The listing builds one solid part. Answer for the finished solid, in the listing's coordinates (mm). Face numbers are marked on the shaded views. Round coordinates to 2 decimals unless told otherwise and drop trailing zeros. Order: outer loops, then holes, each group sorted by start corner. A loop starts at its lowest first (then second) coordinate and runs counter-clockwise, first axis right, second up. Notation, with made-up numbers: (22, -5.5) - (51, -5.5) arc R18 ccw to (51, 21.5) - close; hole circle Ø7 at (51, -30.75). An arc over 180 degrees is marked (long way). One line per item, written item: value. Start each with the question number.
1. Section A-A, the plane z = 0 is taken. Give the vertices of the cut face in (x, y), then the cut area to 3 significant figures.
2. Straight lines are drawn through the part: line 1 (X direction, y = 0.2, z = 0.25); line 2 (Z direction, x = 10, y = 1.25); line 3 (X direction, y = 1.8, z = 10). For each, find the intervals that lie inside material, in ascending order.
3. Section C-C, the plane z = -10 is taken. Give the vertices of the cut face in (x, y), then the cut area to 3 significant figures.
4. Section B-B, the plane x = 10 is taken. Give the vertices of the cut face in (y, z), then the cut area to 3 significant figures.
5. Section D-D, the plane y = 0.5 is taken. Give the vertices of the cut face in (x, z).
6. Flat-ended cylindrical pins translate along their axes: P1, Ø1.3, axis at x = 10, z = 0, coming from the -Y side; P2, Ø0.6, axis at y = 1, z = 8.5, coming from the -X side. Find the tip coordinate at first contact, or state that the pin passes through.
7. For a pull along Z with two mould halves and no side action, classify the marked faces 1, 2, 3 and 4 as released by +Z, released by -Z, zero draft, split by the parting line, or undercut.
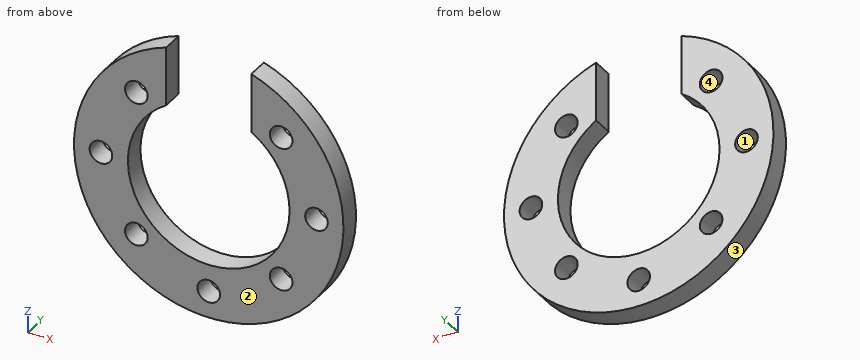
from build123d import *

# Parameters (mm, degrees)
SKETCH1_R           = 12.5
SKETCH1_R_2         = 7.5
BOSS_EXTRUDE1_DEPTH = 2
SKETCH2_R           = 1.05
CUT_EXTRUDE1_DEPTH  = 5
CIRPATTERN1_COUNT   = 3
CIRPATTERN1_ANGLE   = 180
SKETCH3_R           = 1.05
CUT_EXTRUDE2_DEPTH  = 2
SKETCH4_W           = 7.9
SKETCH4_H           = 11.346310676
CUT_EXTRUDE3_DEPTH  = 10


with BuildPart() as part:
    # Sketch1 → Boss-Extrude1 (new body)
    with BuildSketch(Plane(origin=(0, 0, 0), x_dir=(1, 0, 0), z_dir=(0, 1, 0))):
        Circle(SKETCH1_R)
        Circle(SKETCH1_R_2, mode=Mode.SUBTRACT)
    extrude(amount=BOSS_EXTRUDE1_DEPTH)

    # Sketch2 → Cut-Extrude1 (cut)
    with BuildSketch(Plane(origin=(0, 2, 0), x_dir=(1, 0, 0), z_dir=(0, 1, 0))):
        with Locations((10, 0)):
            Circle(SKETCH2_R)
    cut_extrude1 = extrude(amount=-CUT_EXTRUDE1_DEPTH, mode=Mode.SUBTRACT)

    # CirPattern1: Cut-Extrude1 ×3 about axis
    cirpattern1_axis = Axis((0, 0, 0), (0, 1, 0))
    for i in range(1, CIRPATTERN1_COUNT):
        add(cut_extrude1.rotate(cirpattern1_axis, i * CIRPATTERN1_ANGLE / (CIRPATTERN1_COUNT - 1)), mode=Mode.SUBTRACT)

    # Sketch3 → Cut-Extrude2 (cut)
    with BuildSketch(Plane(origin=(0, 2, 0), x_dir=(1, 0, 0), z_dir=(0, 1, 0))):
        with Locations((-6.71751442, 6.71751442)):
            Circle(SKETCH3_R)
        with Locations((6.71751442, 6.71751442)):
            Circle(SKETCH3_R)
        with Locations((6.71751442, -6.71751442)):
            Circle(SKETCH3_R)
        with Locations((-6.71751442, -6.71751442)):
            Circle(SKETCH3_R)
    extrude(amount=-CUT_EXTRUDE2_DEPTH, mode=Mode.SUBTRACT)

    # Sketch4 → Cut-Extrude3 (cut)
    with BuildSketch(Plane(origin=(0, 2, 0), x_dir=(1, 0, 0), z_dir=(0, 1, 0))):
        with Locations((0, -10.263253748)):
            Rectangle(SKETCH4_W, SKETCH4_H)
    extrude(amount=-CUT_EXTRUDE3_DEPTH, mode=Mode.SUBTRACT)


solid = part.part
Answer list:
1. outline: (-12.5, 0) - (-11.05, 0) - (-11.05, 2) - (-12.5, 2) - close; (-8.95, 0) - (-7.5, 0) - (-7.5, 2) - (-8.95, 2) - close; (7.5, 0) - (8.95, 0) - (8.95, 2) - (7.5, 2) - close; (11.05, 0) - (12.5, 0) - (12.5, 2) - (11.05, 2) - close
1. area: 11.6 mm²
2. line 1: x = -12.5 to -11.02, -8.98 to -7.5, 7.5 to 8.98, 11.02 to 12.5
2. line 2: z = -7.5 to -1.05, 1.05 to 7.5
2. line 3: x = -7.5 to -3.95, 3.95 to 7.5
3. outline: (-7.5, 0) - (-1.05, 0) - (-1.05, 2) - (-7.5, 2) - close; (1.05, 0) - (7.5, 0) - (7.5, 2) - (1.05, 2) - close
3. area: 25.8 mm²
4. outline: (0, -7.5) - (2, -7.5) - (2, -1.05) - (0, -1.05) - close; (0, 1.05) - (2, 1.05) - (2, 7.5) - (0, 7.5) - close
4. area: 25.8 mm²
5. outline: (-3.95, 6.38) - (-3.95, 11.86) arc R12.5 ccw (long way) to (3.95, 11.86) - (3.95, 6.38) arc R7.5 cw (long way) to start; hole circle Ø2.1 at (-10, 0); hole circle Ø2.1 at (-6.72, -6.72); hole circle Ø2.1 at (-6.72, 6.72); hole circle Ø2.1 at (0, -10); hole circle Ø2.1 at (6.72, -6.72); hole circle Ø2.1 at (6.72, 6.72); hole circle Ø2.1 at (10, 0)
6. P1: passes through
6. P2: stops at x = -9.43
7. face 1: undercut
7. face 2: zero draft
7. face 3: split by the parting line
7. face 4: undercut
